Design review of the part built by this model. Coordinates are the model's own, in mm. Face numbers are marked on the shaded views. A direction names the side the tool comes from. Coordinates: 2 decimals unless noted, no trailing zeros. Order: outer loops, then holes, each group sorted by start corner. A loop starts at its lowest first (then second) coordinate and runs counter-clockwise, first axis right, second up. Notation, with made-up numbers: (-8.75, -17.5) -> (45.25, -17.5) arc R24 ccw to (45.25, 11.5) -> close; hole circle Ø3 at (34.5, 86). An arc over 180 degrees is marked (long way). Write item = value, one per line.
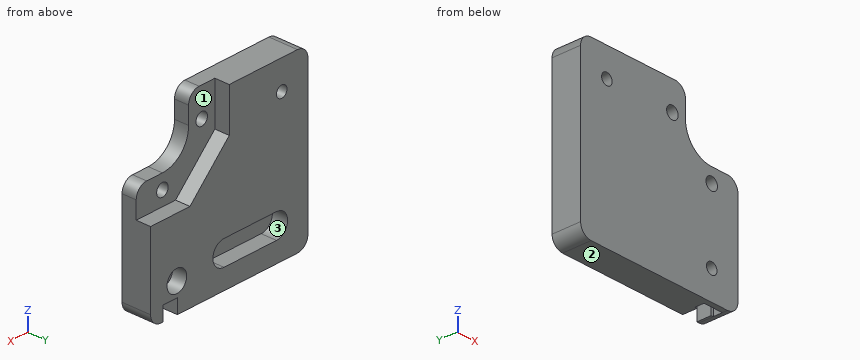
```python
from build123d import *

# Parameters (mm, degrees)
SKETCH1_R           = 2.2
BOSS_EXTRUDE1_DEPTH = 10.1
CUT_EXTRUDE2_DEPTH  = 5.4
CUT_EXTRUDE4_DEPTH  = 5.1
SKETCH9_R           = 2
CUT_EXTRUDE5_DEPTH  = 73.814902321
SKETCH10_R          = 3.75
CUT_EXTRUDE6_DEPTH  = 5
FILLET2_R           = 10
FILLET3_R           = 4
CUT_EXTRUDE7_DEPTH  = 5


with BuildPart() as part:
    # Sketch1 → Boss-Extrude1 (new body)
    with BuildSketch(Plane(origin=(0, 0, 0), x_dir=(1, 0, 0), z_dir=(0, 1, 0))):
        Polygon((0, 0), (0, 20), (20, 20), (20, 60), (-40, 60), (-40, 0), align=None)
        with Locations(Location((10, 25, 0), (0, 0, 270))):
            Circle(SKETCH1_R, mode=Mode.SUBTRACT)
        with Locations(Location((-5, 10, 0), (0, 0, 90))):
            Circle(SKETCH1_R, mode=Mode.SUBTRACT)
    extrude(amount=BOSS_EXTRUDE1_DEPTH)

    # Sketch4 → Cut-Extrude2 (cut)
    with BuildSketch(Plane(origin=(0, 10.1, 0), x_dir=(1, 0, 0), z_dir=(0, 1, 0))):
        with BuildLine():
            Line((-28, 53.083248844), (-8, 53.083248844))
            ThreePointArc((-8, 53.083248844), (-3.75, 48.833248844), (-8, 44.583248844))
            Line((-8, 44.583248844), (-28, 44.583248844))
            ThreePointArc((-28, 44.583248844), (-32.25, 48.833248844), (-28, 53.083248844))
        make_face()
    extrude(amount=-CUT_EXTRUDE2_DEPTH, mode=Mode.SUBTRACT)

    # Sketch7 → Cut-Extrude4 (cut)
    with BuildSketch(Plane(origin=(0, 10.1, 0), x_dir=(1, 0, 0), z_dir=(0, 1, 0))):
        Polygon((20, 0), (-10, 0), (-10, 15), (5, 30), (20, 30), align=None)
    extrude(amount=-CUT_EXTRUDE4_DEPTH, mode=Mode.SUBTRACT)

    # Sketch9 → Cut-Extrude5 (cut, through all)
    with BuildSketch(Plane(origin=(0, 10.1, 0), x_dir=(1, 0, 0), z_dir=(0, 1, 0))):
        with Locations(Location((-30, 10, 0), (0, 0, 270))):
            Circle(SKETCH9_R)
        with Locations(Location((10, 50, 0), (0, 0, 90))):
            Circle(SKETCH9_R)
    extrude(amount=-CUT_EXTRUDE5_DEPTH, mode=Mode.SUBTRACT)

    # Sketch10 → Cut-Extrude6 (cut)
    with BuildSketch(Plane(origin=(0, 10.1, 0), x_dir=(1, 0, 0), z_dir=(0, 1, 0))):
        with Locations(Location((10, 50, 0), (0, 0, 270))):
            Circle(SKETCH10_R)
    extrude(amount=-CUT_EXTRUDE6_DEPTH, mode=Mode.SUBTRACT)

    # Fillet2
    fillet2_edges = [part.edges().sort_by_distance(p)[0] for p in [
        (0, 2.5, -20),
    ]]
    fillet(fillet2_edges, radius=FILLET2_R)

    # Fillet3
    fillet3_edges = [part.edges().sort_by_distance(p)[0] for p in [
        (-40, 5.05, -60),
        (20, 5.05, -60),
        (-40, 5.05, 0),
        (20, 2.5, -20),
        (0, 2.5, 0),
    ]]
    fillet(fillet3_edges, radius=FILLET3_R)

    # Sketch11 → Cut-Extrude7 (cut)
    with BuildSketch(Plane(origin=(0, 0, -60), x_dir=(-1, 0, 0), z_dir=(0, 0, -1))):
        Polygon((-16, 5), (-15.2, 5), (-15.2, 10.1), (-9.8, 10.1), (-9.8, 5), (-9, 5), (-9, 1.8), (-16, 1.8), align=None)
    extrude(amount=-CUT_EXTRUDE7_DEPTH, mode=Mode.SUBTRACT)


solid = part.part
```
(1) We need section D-D (x = -30). Write out the cut boundary in (y, z), and give its area (3 significant figures).
Report:
outline = (0, -60) -> (10.1, -60) -> (10.1, -52.58) -> (4.7, -52.58) -> (4.7, -45.08) -> (10.1, -45.08) -> (10.1, -12) -> (0, -12) -> close; (0, -8) -> (10.1, -8) -> (10.1, 0) -> (0, 0) -> close
area = 525 mm²
(2) We need section A-A (z = -25). Write out the cut boundary in (x, y), and give its area (3 significant figures).
Report:
outline = (-40, 0) -> (7.8, 0) -> (7.8, 5) -> (0, 5) -> (0, 10.1) -> (-40, 10.1) -> close; (12.2, 0) -> (20, 0) -> (20, 5) -> (12.2, 5) -> close
area = 482 mm²
(3) We need section C-C (x = -9). Write out the cut boundary in (y, z).
Report:
outline = (0, -60) -> (10.1, -60) -> (10.1, -53.08) -> (4.7, -53.08) -> (4.7, -44.58) -> (10.1, -44.58) -> (10.1, -16) -> (5, -16) -> (5, 0) -> (0, 0) -> close
(4) Insertion check: pin 1 (5.5 mm diameter, centred on y = 6.5, z = -8.5, fed in from +X); pin 2 (6 mm diameter, centred on y = 9, z = -8.5, fed in from +X); pin 3 (4 mm diameter, centred on x = 13, z = -57.5, fed in from +Y). Each pin has a flat end and moves straight along its axis. Give the tip position at first contact, or say it passes through.
Report:
pin_1 = 0.03
pin_2 = -10
pin_3 = 1.8
(5) For the marked faces 1, 2 and 3, list the 3-axis set-ups (+Z, -Z, +X, -X, +Y, -Y) from which the entire face can be reached by the end or side of a thin tool; tool diameter is ignored.
Report:
face_1 = +Z, +X, +Y
face_2 = -Z, +X, -X, +Y, -Y
face_3 = +Y
(6) We need section B-B (y = 3.5). Write out the cut boundary in (x, z), and give its area (3 significant figures).
Report:
outline = (-40, -56) arc R4 ccw to (-36, -60) -> (9, -60) -> (9, -55) -> (16, -55) -> (16, -60) arc R4 ccw to (20, -56) -> (20, -24) arc R4 ccw to (16, -20) -> (10, -20) arc R10 cw to (0, -10) -> (0, -4) arc R4 ccw to (-4, 0) -> (-36, 0) arc R4 ccw to (-40, -4) -> close; hole circle Ø4 at (-30, -10); hole circle Ø4.4 at (-5, -10); hole circle Ø4.4 at (10, -25); hole circle Ø4 at (10, -50)
area = 3,110 mm²
(7) For L1, parallel to Z at x = 10, y = 3.3; L2, parallel to Z at x = 10, y = 1.5; L3, parallel to X at y = 3.1, z = -25, list the stretches that pass through material, from the lowest coordinate up.
Report:
L1 = -55 to -52, -48 to -27.2, -22.8 to -20
L2 = -60 to -52, -48 to -27.2, -22.8 to -20
L3 = -40 to 7.8, 12.2 to 20
